Source: CAD feature listing. Evaluate the final solid. Frame: model axes, mm. A direction names the side the tool comes from. Give positions to 0.01 mm unless a question says otherwise; leave off trailing zeros. Write item = value, one per line.
from build123d import *

# Parameters (mm, degrees)
BOSS_EXTRUDE1_DEPTH = 80
SKETCH2_R           = 1.5
CUT_EXTRUDE1_DEPTH  = 11
SKETCH3_R           = 4.5
CUT_EXTRUDE2_DEPTH  = 2
SKETCH4_R           = 1.5
CUT_EXTRUDE3_DEPTH  = 10
SKETCH6_R           = 4.5
CUT_EXTRUDE4_DEPTH  = 2
LPATTERN1_COUNT     = 8
LPATTERN1_PITCH     = 10
LPATTERN2_COUNT     = 7
LPATTERN2_PITCH     = 10


with BuildPart() as part:
    # Sketch1 → Boss-Extrude1 (new body)
    with BuildSketch(Plane.XY):
        Polygon((-10, 0), (-10, -3.55), (-11, -3.55), (-11, -6.45), (-10, -6.45), (-10, -10), (0, -10), (0, 0), align=None)
    extrude(amount=BOSS_EXTRUDE1_DEPTH)

    # Sketch2 → Cut-Extrude1 (cut, through all)
    with BuildSketch(Plane(origin=(0, 0, 0), x_dir=(1, 0, 0), z_dir=(0, 1, 0))):
        with Locations((-5, -75)):
            Circle(SKETCH2_R)
    cut_extrude1 = extrude(amount=-CUT_EXTRUDE1_DEPTH, mode=Mode.SUBTRACT)

    # Sketch3 → Cut-Extrude2 (cut)
    with BuildSketch(Plane(origin=(0, 0, 0), x_dir=(0, 0, -1), z_dir=(1, 0, 0))):
        with Locations((-70, -5)):
            Circle(SKETCH3_R)
    cut_extrude2 = extrude(amount=-CUT_EXTRUDE2_DEPTH, mode=Mode.SUBTRACT)

    # Sketch4 → Cut-Extrude3 (cut, through all)
    with BuildSketch(Plane(origin=(-2, 0, 0), x_dir=(0, 0, -1), z_dir=(1, 0, 0))):
        with Locations((-70, -5)):
            Circle(SKETCH4_R)
    cut_extrude3 = extrude(amount=-CUT_EXTRUDE3_DEPTH, mode=Mode.SUBTRACT)

    # Sketch6 → Cut-Extrude4 (cut)
    with BuildSketch(Plane(origin=(0, 0, 0), x_dir=(1, 0, 0), z_dir=(0, 1, 0))):
        with Locations((-5, -75)):
            Circle(SKETCH6_R)
    cut_extrude4 = extrude(amount=-CUT_EXTRUDE4_DEPTH, mode=Mode.SUBTRACT)

    # LPattern1: Cut-Extrude1, Cut-Extrude4 ×8
    with Locations(*[(0, 0, -i * LPATTERN1_PITCH) for i in range(1, LPATTERN1_COUNT)]):
        add(cut_extrude1, mode=Mode.SUBTRACT)
        add(cut_extrude4, mode=Mode.SUBTRACT)

    # LPattern2: Cut-Extrude2, Cut-Extrude3 ×7
    with Locations(*[(0, 0, -i * LPATTERN2_PITCH) for i in range(1, LPATTERN2_COUNT)]):
        add(cut_extrude2, mode=Mode.SUBTRACT)
        add(cut_extrude3, mode=Mode.SUBTRACT)


solid = part.part
1. Reachability of faces 1 (the flat face through (-10, -2, 39)), 2 (the cylindrical face through (-0.99, -8.99, 17.92)), 3 (the flat face through (-5, -2, 67)), 4 (the cylindrical face through (-6.2, -5.9, 35.9)) from +Z, -Z, +X, -X, +Y, -Y: full face, straight path, thin tool, end or side. Return the list, or none.
Derived:
face_1 = +Z, -Z, -X, +Y
face_2 = +X
face_3 = +Y
face_4 = +Y, -Y
2. Cut plane A-A, the plane x = -5.5. Count the separate pieces of the cut face and the enclosed holes in it, then the cut area to 3 significant figures.
Derived:
separate_pieces = 9
enclosed_holes = 7
area = 426 mm²
3. Pull-direction query (Z, two-part tool) for faces 5 (the cylindrical face through (-4.31, -5.94, 46.33)), 6 (the flat face through (-11, -5, 75)); classes: +Z half, -Z half, draft (parallel to the pull), parting line (faces both ways), or undercut.
Derived:
face_5 = undercut
face_6 = draft
4. Material intervals for probe 1 along X at (y, z) = (-7, 25); probe 2 along X at (y, z) = (-0.6, 5), sorted ascending. Write a range as from..to.
Derived:
probe_1 = -10..-6.5, -3.5..0
probe_2 = -10..-9.5, -0.5..0
5. First-contact query: pin 1 Ø0.5 at (x, z) = (-10.5, 13.5) entering from -Y; pin 2 Ø5.5 at (x, z) = (-5, 55) entering from +Y; pin 3 Ø4 at (y, z) = (-8, 70.5) entering from -X; pin 4 Ø2.5 at (y, z) = (-7, 22) entering from +X. Flat tips, straight axial feed; report the tip coordinate or a pass-through.
Derived:
pin_1 = -6.45
pin_2 = -2
pin_3 = -11
pin_4 = -2
